Job drawing, mm, ordinate dimensions from the low corner. One solid piece. Give positions to 0.01 mm unless a question says otherwise; leave off trailing zeros. Order: outer loops, then holes, each group sorted by start corner. A loop starts at its lowest first (then second) coordinate and runs counter-clockwise, first axis right, second up. Notation, with made-up numbers: (-30.75, 65) - (-18.75, 65) arc R33 cw to (-18.75, 103) - close; hole circle Ø2 at (79, -22). An arc over 180 degrees is marked (long way). Use a Markdown table: item, result. Add a question column.
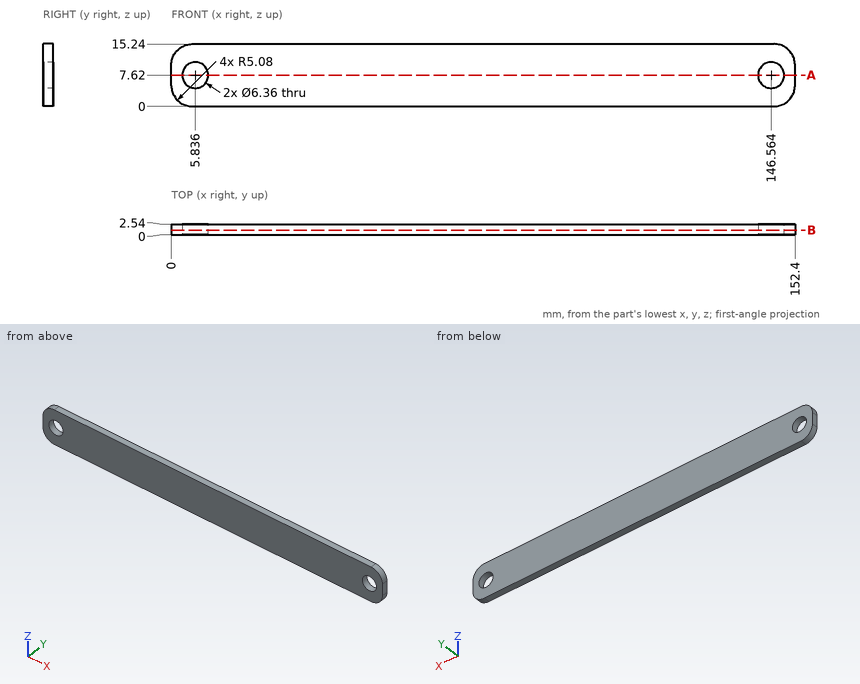
1. Drill centre lines: probe 1 along X at (y, z) = (1.55, 7.75); probe 2 along X at (y, z) = (0.6, 4.75) (1 decimal); probe 3 along Z at (x, y) = (144, 2.4). Where is each one in solid material? Low to high. Write a range as [from, to].
2. Cut at A-A (z = 7.62). Write the cut outline in (x, y), plus the area to 3 significant figures.
3. Cut at B-B (y = 1.1). Write the cut outline in (x, z), plus the area to 3 significant figures.
4. Pin check, flat tip, straight feed: P1, Ø5.5, axis at x = 5.84, z = 7.62, coming from the +Y side. Stop position of the tip, or through.
Responses:
| question | item | result |
|---|---|---|
| 1 | probe 1 | x = [0, 2.66], [9.01, 143.39], [149.74, 152.4] |
| 1 | probe 2 | x = [0, 4.5], [7.2, 145.2], [147.9, 152.4] |
| 1 | probe 3 | z = [0, 5.74], [9.5, 15.24] |
| 2 | outline | (0, 0) - (2.66, 0) - (2.66, 2.54) - (0, 2.54) - close; (9.02, 0) - (143.38, 0) - (143.38, 2.54) - (9.02, 2.54) - close; (149.74, 0) - (152.4, 0) - (152.4, 2.54) - (149.74, 2.54) - close |
| 2 | area | 355 mm² |
| 3 | outline | (0, 5.08) arc R5.08 ccw to (5.08, 0) - (147.32, 0) arc R5.08 ccw to (152.4, 5.08) - (152.4, 10.16) arc R5.08 ccw to (147.32, 15.24) - (5.08, 15.24) arc R5.08 ccw to (0, 10.16) - close; hole circle Ø6.36 at (5.84, 7.62); hole circle Ø6.36 at (146.56, 7.62) |
| 3 | area | 2,240 mm² |
| 4 | P1 | passes through |
